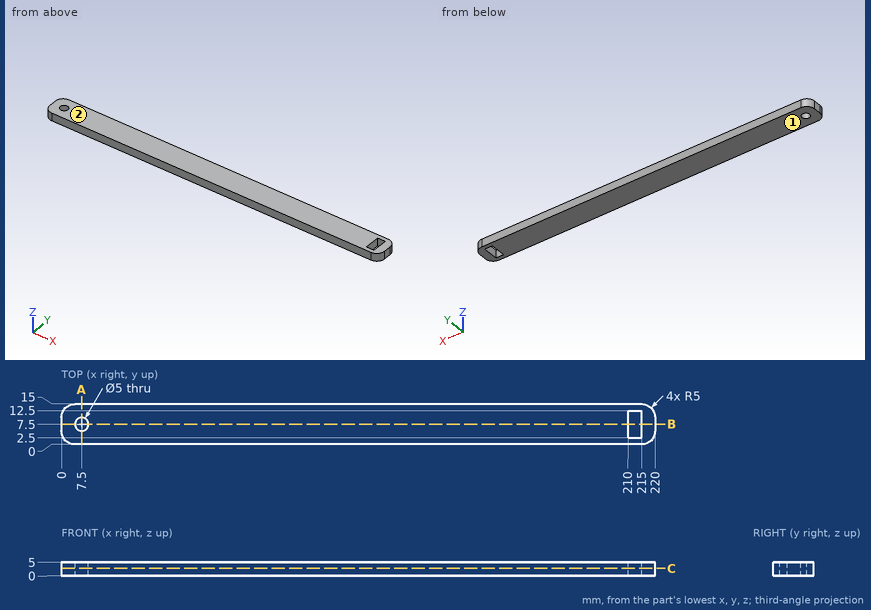
Job drawing, mm, ordinate dimensions from the low corner. One solid piece. Give positions to 0.01 mm unless a question says otherwise; leave off trailing zeros. Write each loop counter-clockwise with the first axis right and the second up, starting at its lowest first coordinate (ties: lowest second). Pieces come first, ordered by that corner, then holes. Notation, with made-up numbers: M 2,38 L 56,38 A13 cw 56,43 Z; hole C 0.5,-8.5 d3. An arc over 180 degrees is marked long. Put each result on its own line as item: value. Start each with the question number.
(1) Mould opens along Z. For the marked faces 1 and 2 say: +Z half, -Z half, draft (parallel to the pull), parting line (faces both ways), or undercut.
(2) Band-saw the part on A-A, the plane x = 7.5. Write the cut outline in (y, z), and give its area (3 significant figures).
(3) Band-saw the part on C-C, the plane z = 2.8. Write the cut outline in (x, y).
(4) Flat gauge pins, fed straight in: pin 1 Ø6 at (x, y) = (7.5, 7.5) entering from -Z; pin 2 Ø1 at (y, z) = (11, 1.5) entering from -X; pin 3 Ø1.5 at (y, z) = (11, 1.5) entering from +X. Where does each tip first touch, or does it go through?
(5) Probe L1, parallel to Y at x = 7.5, z = 3.8; L2, parallel to X at y = 4.5, z = 2.8; L3, parallel to X at y = 3.5, z = 2.5. List the from-to ranges inside material, lowest first.
(6) Band-saw the part on B-B, the plane y = 7.5. Write the cut outline in (x, z), and give its area (3 significant figures).
Response values:
1. face 1: -Z half
1. face 2: +Z half
2. outline: M 0,0 L 5,0 L 5,5 L 0,5 Z; M 10,0 L 15,0 L 15,5 L 10,5 Z
2. area: 50.0 mm2
3. outline: M 0,5 A5 ccw 5,0 L 215,0 A5 ccw 220,5 L 220,10 A5 ccw 215,15 L 5,15 A5 ccw 0,10 Z; hole C 7.5,7.5 d5; hole M 210,2.5 L 215,2.5 L 215,12.5 L 210,12.5 Z
4. pin 1: stops at z = 0
4. pin 2: stops at x = 0.03
4. pin 3: stops at x = 219.99
5. L1: y = 0 to 5, 10 to 15
5. L2: x = 0.03 to 210, 215 to 219.97
5. L3: x = 0.23 to 210, 215 to 219.77
6. outline: M 0,0 L 5,0 L 5,5 L 0,5 Z; M 10,0 L 210,0 L 210,5 L 10,5 Z; M 215,0 L 220,0 L 220,5 L 215,5 Z
6. area: 1,050 mm2
